Part model, mm, in its own coordinate system. Face numbers are marked on the shaded views. Round coordinates to 2 decimals unless told otherwise and drop trailing zeros. Loops run counter-clockwise (first coordinate to the right, second up) from the corner with the lowest first, then second, coordinate; pieces in that order, holes last. Notation, with made-up numbers: (-28.5, 78.5) - (2.5, 78.5) arc R9 cw to (2.5, 86.5) - close; hole circle Ø11 at (26.5, 59). An arc over 180 degrees is marked (long way). Put each result on its own line as item: value.
from build123d import *

# Parameters (mm, degrees)
M3_CLEARANCE_HOLE1_D = 3.6
CHAMFER1_SIZE        = 0.8


with BuildPart() as part:
    # Sketch1 → Revolve1 (revolve)
    with BuildSketch(Plane.XY, mode=Mode.PRIVATE) as revolve1_sk:
        Polygon((-25.75, 0), (-27.5, 0), (-27.5, 10), (-13.25, 10), (-13.25, 7.5), (-16.25, 7.5), (-16.25, 5), (-19.25, 5), (-19.25, 7), (-25.75, 7), align=None)
    revolve(revolve1_sk.sketch.rotate(Axis((0, 0, 0), (0, -1, 0)), 270), axis=Axis((0, 0, 0), (0, -1, 0)))

    # M3 Clearance Hole1 (through all)
    with Locations(Plane(origin=(0, 10, 0), x_dir=(1, 0, 0), z_dir=(0, 1, 0))):
        with Locations((-22.5, 0), (-19.485571585, 11.25), (-11.25, 19.485571585), (0, 22.5), (11.25, 19.485571585), (19.485571585, 11.25), (22.5, 0), (19.485571585, -11.25), (11.25, -19.485571585), (0, -22.5), (-11.25, -19.485571585), (-19.485571585, -11.25)):
            Hole(M3_CLEARANCE_HOLE1_D / 2)

    # Chamfer1
    chamfer1_edges = [part.edges().sort_by_distance(p)[0] for p in [
        (0, 7.5, -13.25),
        (0, 5, -16.25),
    ]]
    chamfer(chamfer1_edges, length=CHAMFER1_SIZE)


solid = part.part
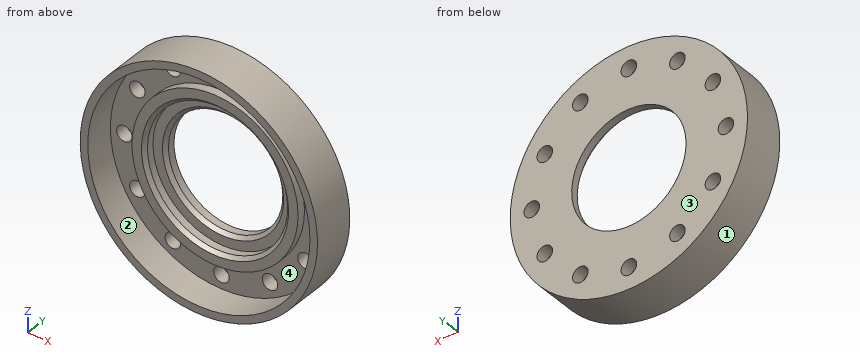
1. Band-saw the part on B-B (x = 22.5). List the corners of the cut face in (y, z).
A:
outline: (0, -15.81) - (10, -15.81) - (10, -1.8) - (7, -1.8) - (7, -12.52) - (0, -12.52) - close; (0, 12.52) - (7, 12.52) - (7, 1.8) - (10, 1.8) - (10, 15.81) - (0, 15.81) - close
2. Two-plate mould, pull along Z, no slides. Class the marked faces 1, 2, 3 and 4: pulls with the +Z half, pulls with the -Z half, needs draft (parallel to the pull), parting line crosses it, or undercut.
A:
face 1: parting line crosses it
face 2: undercut
face 3: needs draft
face 4: undercut
3. Band-saw the part on A-A (z = 0). Give the number of separate pieces and of enclosed holes in the cut face, plus the area to 3 significant figures.
A:
separate pieces: 4
enclosed holes: 0
area: 96.1 mm²
4. Pin check, flat tips, straight feed: P1, Ø1, axis at x = 3, y = 5.5, coming from the +Z side; P2, Ø5, axis at x = -8.5, y = 6.5, coming from the +Z side; P3, Ø4, axis at x = 19, y = 6.5, coming from the +Z side. Stop position of each tip, or through.
A:
P1: stops at z = 27.39
P2: stops at z = 26.84
P3: stops at z = 21.62
5. Probe line 1 along Z through (x, y) = (10, 8.25); line 2 along X through (y, z) = (5.75, 14); line 3 along X through (y, z) = (8.2, -11.25). List the from-to ranges inside material, lowest first. Write a range as [from, to].
A:
line 1: z = [-25.62, -20.78], [-18.19, -8.77], [8.77, 18.19], [20.78, 25.62]
line 2: x = [-23.67, -21.61], [-13.21, -8.35], [8.35, 13.21], [21.61, 23.67]
line 3: x = [-25.09, -21.29], [-17.69, -7.19], [7.19, 17.69], [21.29, 25.09]
6. Band-saw the part on D-D (y = 2.25). List the corners of the cut face in (x, z).
A:
outline: circle Ø55 at (0, 0); hole circle Ø51.5 at (0, 0)
7. Band-saw the part on C-C (z = 22.5). List the corners of the cut face in (x, y).
A:
outline: (-15.81, 0) - (-12.52, 0) - (-12.52, 7) - (-1.8, 7) - (-1.8, 10) - (-15.81, 10) - close; (1.8, 7) - (12.52, 7) - (12.52, 0) - (15.81, 0) - (15.81, 10) - (1.8, 10) - close
